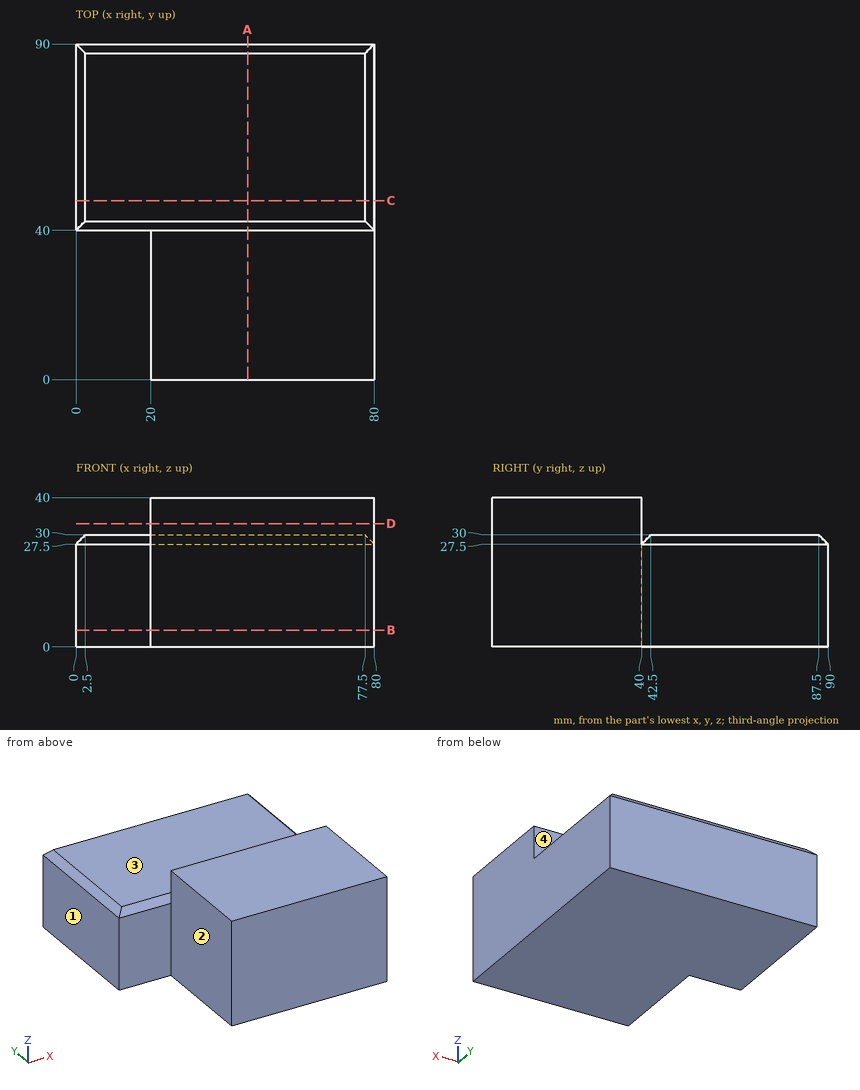
Here's the drawing with two shaded views (mm, measured from the low corner). I have some questions. A direction names the side the tool comes from. Give positions to 0.01 mm unless a question says otherwise; leave off trailing zeros. Write each loop counter-clockwise with the first axis right and the second up, starting at its lowest first coordinate (ties: lowest second). Pieces come first, ordered by that corner, then holes. Notation, with made-up numbers: (84, 44) -> (99, 44) arc R23 ccw to (99, 63) -> close; hole circle Ø6 at (4, 32). An arc over 180 degrees is marked (long way). Use one line per item in the form item = value.
1) Suppose I cut it at C-C (y = 48). Please give me the cut outline in (x, z), and give its area (3 significant figures).
Verdict:
outline = (0, 0) -> (80, 0) -> (80, 27.5) -> (77.5, 30) -> (2.5, 30) -> (0, 27.5) -> close
area = 2,390 mm2
2) On a 3-axis mill with a long thin cutter (end or side, diameter ignored), from which of +Z, -Z, +X, -X, +Y, -Y can I reach the whole of each face in a straight line? I mean the marked faces 1, 2, 3 and 4. Say none if no direction works.
Verdict:
face_1 = +Z, -Z, -X, +Y, -Y
face_2 = +Z, -Z, -X, -Y
face_3 = +Z, +X, -X, +Y
face_4 = +Z, +X, -X
3) Suppose I cut it at D-D (z = 33). Please give me the cut outline in (x, y).
Verdict:
outline = (20, 0) -> (80, 0) -> (80, 40) -> (20, 40) -> close
4) If I drill on L1, parallel to Z at x = 52.5, y = 49; L2, parallel to X at y = 19.5, z = 34; L3, parallel to Y at x = 19, z = 10, over which ranges is the centre line in solid material (lowest first)? Write a range as [from, to].
Verdict:
L1 = [0, 30]
L2 = [20, 80]
L3 = [40, 90]
5) Suppose I cut it at A-A (x = 46). Please give me the cut outline in (y, z), and give its area (3 significant figures).
Verdict:
outline = (0, 0) -> (90, 0) -> (90, 27.5) -> (87.5, 30) -> (42.5, 30) -> (40, 27.5) -> (40, 40) -> (0, 40) -> close
area = 3,090 mm2
6) Suppose I cut it at B-B (z = 4.5). Please give me the cut outline in (x, y), and give its area (3 significant figures).
Verdict:
outline = (0, 40) -> (20, 40) -> (20, 0) -> (80, 0) -> (80, 90) -> (0, 90) -> close
area = 6,400 mm2
7) I'm going to push flat-ended pins straight in: pin 1 (2 mm diameter, centred on x = 26, y = 31, fed in from -Z); pin 2 (4 mm diameter, centred on x = 40, z = 33.5, fed in from +Y); pin 3 (22.5 mm diameter, centred on x = 31, y = 56, fed in from +Z); pin 4 (10 mm diameter, centred on y = 28.5, z = 7.5, fed in from -X). Where does each tip first touch, or does it pass through?
Verdict:
pin_1 = 0
pin_2 = 40
pin_3 = 30
pin_4 = 20
